Source: CAD feature listing. Evaluate the final solid. Frame: model axes, mm. Face numbers are marked on the shaded views. A direction names the side the tool comes from. Give positions to 0.01 mm unless a question says otherwise; leave off trailing zeros. Write each loop counter-clockwise with the first axis right and the second up, starting at its lowest first coordinate (ties: lowest second). Pieces come first, ordered by that corner, then holes. Notation, with made-up numbers: (-34, 26) -> (10, 26) arc R4 ccw to (10, 31) -> close; hole circle Ø3 at (89.25, 87). An arc over 180 degrees is marked (long way). Write item = value, one per line.
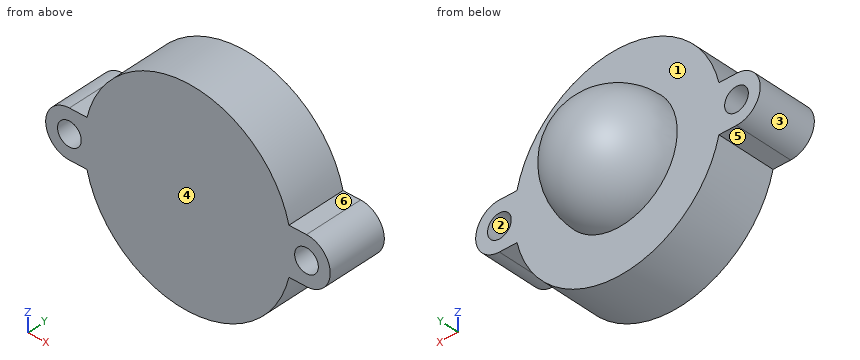
from build123d import *

# Parameters (mm, degrees)
SKETCH1_R           = 17.5
SKETCH1_R_2         = 2
BOSS_EXTRUDE1_DEPTH = 10
REVOLVE1_ANGLE      = 180


with BuildPart() as part:
    # Sketch1 → Boss-Extrude1 (new body)
    # profile 1 of 2: a face of its own
    with BuildSketch(Plane(origin=(0, 0, 0), x_dir=(1, 0, 0), z_dir=(0, 1, 0))):
        Circle(SKETCH1_R)
    # profile 2 of 2: a face of its own
    with BuildSketch(Plane(origin=(0, 0, 0), x_dir=(1, 0, 0), z_dir=(0, 1, 0))):
        with BuildLine():
            Line((-20, -4), (20, -4))
            ThreePointArc((20, -4), (24, 0), (20, 4))
            Line((20, 4), (-20, 4))
            ThreePointArc((-20, 4), (-24, 0), (-20, -4))
        make_face()
        with Locations(Location((-20, 0, 0), (0, 0, 270))):
            Circle(SKETCH1_R_2, mode=Mode.SUBTRACT)
        with Locations(Location((20, 0, 0), (0, 0, 270))):
            Circle(SKETCH1_R_2, mode=Mode.SUBTRACT)
    extrude(amount=BOSS_EXTRUDE1_DEPTH)

    # Sketch2 → Revolve1 (revolve)
    with BuildSketch(Plane(origin=(0, 10, 0), x_dir=(1, 0, 0), z_dir=(0, 1, 0))):
        with BuildLine():
            Line((0, 10), (0, -10))
            ThreePointArc((0, -10), (-10, 0), (0, 10))
        make_face()
    revolve(axis=Axis((0, 10, -10), (0, 0, -1)), revolution_arc=REVOLVE1_ANGLE)


solid = part.part
1) Material intervals for L1, parallel to X at y = 4.5, z = 0; L2, parallel to Z at x = 19.5, y = 8.25; L3, parallel to Y at x = 15.5, z = 5, sorted ascending.
Computed:
L1 = -24 to -22, -18 to 18, 22 to 24
L2 = -4 to -1.94, 1.94 to 4
L3 = 0 to 10
2) Cut plane A-A (z = 0). Return the cut outline in (x, y), then the cut area to 3 significant figures.
Computed:
outline = (-24, 0) -> (-22, 0) -> (-22, 10) -> (-24, 10) -> close; (-18, 0) -> (18, 0) -> (18, 10) -> (10, 10) arc R10 ccw to (-10, 10) -> (-18, 10) -> close; (22, 0) -> (24, 0) -> (24, 10) -> (22, 10) -> close
area = 557 mm²
3) Draft query along Z for the marked faces 1, 2 and 3. Return one class per face: pulls with the +Z half, pulls with the -Z half, needs draft (parallel to the pull), parting line crosses it, or undercut.
Computed:
face_1 = needs draft
face_2 = undercut
face_3 = parting line crosses it
4) Access query for the marked faces 4, 5 and 6. Directions: +Z, -Z, +X, -X, +Y, -Y. A direction counts if a zero-diameter tool reaches every point of the face in a straight line with its end or side. Return the directions, or none.
Computed:
face_4 = +Z, -Z, +X, -X, -Y
face_5 = -Z, -X, +Y, -Y
face_6 = +Z, +X, +Y, -Y
5) Cut plane D-D (z = -13). Return the cut outline in (x, y).
Computed:
outline = (-11.72, 0) -> (11.72, 0) -> (11.72, 10) -> (-11.72, 10) -> close
6) Cut plane C-C (x = 4). Return the cut outline in (y, z), then the cut area to 3 significant figures.
Computed:
outline = (0, -17.04) -> (10, -17.04) -> (10, -9.17) arc R9.17 ccw to (10, 9.17) -> (10, 17.04) -> (0, 17.04) -> close
area = 473 mm²
7) Cut plane B-B (y = 8). Return the cut outline in (x, z), then the cut area to 3 significant figures.
Computed:
outline = (-20, -4) -> (-17.04, -4) arc R17.5 ccw to (17.04, -4) -> (20, -4) arc R4 ccw to (20, 4) -> (17.04, 4) arc R17.5 ccw to (-17.04, 4) -> (-20, 4) arc R4 ccw to start; hole circle Ø4 at (-20, 0); hole circle Ø4 at (20, 0)
area = 1,030 mm²
8) Contact query for flat-ended pins moving along their axis: pin 1 (4 mm diameter, centred on y = 3, z = -4, fed in from -X); pin 2 (0.9 mm diameter, centred on x = -18.5, y = 4.5, fed in from +Z); pin 3 (5 mm diameter, centred on y = 15, z = -2, fed in from +X). Output: stop coordinate, or through.
Computed:
pin_1 = -23.46
pin_2 = 4
pin_3 = 9.57
